Geometry check sheet. Reference: the model listing, model coordinates, mm. A direction names the side the tool comes from. Round coordinates to 2 decimals unless told otherwise and drop trailing zeros. Write each loop counter-clockwise with the first axis right and the second up, starting at its lowest first coordinate (ties: lowest second). Pieces come first, ordered by that corner, then holes. Notation, with made-up numbers: (-15.5, 14) -> (16.5, 14) arc R26 cw to (16.5, 28) -> close; hole circle Ø10 at (-6, 62.5). An arc over 180 degrees is marked (long way). One line per question, with ' | ' between items.
```python
from build123d import *

# Parameters (mm, degrees)
BOSS_EXTRUDE1_DEPTH = 180
SKETCH2_R           = 2.9
CUT_EXTRUDE1_DEPTH  = 4
SKETCH3_R           = 1.7
CUT_EXTRUDE2_DEPTH  = 181.269243078


with BuildPart() as part:
    # Sketch1 → Boss-Extrude1 (new body)
    with BuildSketch(Plane.XY):
        Polygon((9, 6.4), (9, 4.9), (8.2, 4.45), (9, 4), (9, 0), (0, 0), (0, 4), (0.8, 4.45), (0, 4.9), (0, 6.4), align=None)
    extrude(amount=BOSS_EXTRUDE1_DEPTH)

    # Sketch2 → Cut-Extrude1 (cut)
    with BuildSketch(Plane(origin=(0, 6.4, 0), x_dir=(1, 0, 0), z_dir=(0, 1, 0))):
        with Locations(Location((4.5, -170, 0), (0, 0, 270))):
            Circle(SKETCH2_R)
        with Locations(Location((4.5, -150, 0), (0, 0, 270))):
            Circle(SKETCH2_R)
        with Locations(Location((4.5, -130, 0), (0, 0, 270))):
            Circle(SKETCH2_R)
        with Locations(Location((4.5, -110, 0), (0, 0, 270))):
            Circle(SKETCH2_R)
        with Locations(Location((4.5, -90, 0), (0, 0, 270))):
            Circle(SKETCH2_R)
        with Locations(Location((4.5, -70, 0), (0, 0, 270))):
            Circle(SKETCH2_R)
        with Locations(Location((4.5, -50, 0), (0, 0, 270))):
            Circle(SKETCH2_R)
        with Locations(Location((4.5, -30, 0), (0, 0, 270))):
            Circle(SKETCH2_R)
        with Locations(Location((4.5, -10, 0), (0, 0, 270))):
            Circle(SKETCH2_R)
    extrude(amount=-CUT_EXTRUDE1_DEPTH, mode=Mode.SUBTRACT)

    # Sketch3 → Cut-Extrude2 (cut, through all)
    with BuildSketch(Plane(origin=(0, 2.4, 0), x_dir=(1, 0, 0), z_dir=(0, 1, 0))):
        with Locations(Location((4.5, -170, 0), (0, 0, 270))):
            Circle(SKETCH3_R)
        with Locations(Location((4.5, -150, 0), (0, 0, 270))):
            Circle(SKETCH3_R)
        with Locations(Location((4.5, -130, 0), (0, 0, 270))):
            Circle(SKETCH3_R)
        with Locations(Location((4.5, -110, 0), (0, 0, 270))):
            Circle(SKETCH3_R)
        with Locations(Location((4.5, -90, 0), (0, 0, 270))):
            Circle(SKETCH3_R)
        with Locations(Location((4.5, -70, 0), (0, 0, 270))):
            Circle(SKETCH3_R)
        with Locations(Location((4.5, -50, 0), (0, 0, 270))):
            Circle(SKETCH3_R)
        with Locations(Location((4.5, -30, 0), (0, 0, 270))):
            Circle(SKETCH3_R)
        with Locations(Location((4.5, -10, 0), (0, 0, 270))):
            Circle(SKETCH3_R)
    extrude(amount=-CUT_EXTRUDE2_DEPTH, mode=Mode.SUBTRACT)


solid = part.part
```
(1) Access from +Z, -Z, +X, -X, +Y, -Y to the whole of each face (thin tool, end or side, straight path). Record for faces 5 (the cylindrical face through (3.85, 1.22, 131.57)), 6 (the cylindrical face through (5.371, 4.428, 32.766)).
Resolved:
face 5: +Y, -Y | face 6: +Y
(2) Draft check along Z on faces 1 (the flat face through (2.6, 2.4, 70)), 2 (the flat face through (5, 3, 0)), 3 (the flat face through (5, 3, 180)), 4 (the flat face through (2.6, 0, 88.7)). Enter one of: +Z half, -Z half, draft (parallel to the pull), parting line (faces both ways), or undercut.
Resolved:
face 1: undercut | face 2: -Z half | face 3: +Z half | face 4: draft
(3) Sectioned sample at A-A on z = 110. Record the cut outline in (x, y), then the cut area to 3 significant figures.
Resolved:
outline: (0, 0) -> (2.8, 0) -> (2.8, 2.4) -> (1.6, 2.4) -> (1.6, 6.4) -> (0, 6.4) -> (0, 4.9) -> (0.8, 4.45) -> (0, 4) -> close; (6.2, 0) -> (9, 0) -> (9, 4) -> (8.2, 4.45) -> (9, 4.9) -> (9, 6.4) -> (7.4, 6.4) -> (7.4, 2.4) -> (6.2, 2.4) -> close | area: 25.5 mm2
(4) Go/stop test with flat-tipped pins: pin 1 (4 mm diameter, centred on x = 4.5, z = 170, fed in from +Y); pin 2 (1.7 mm diameter, centred on x = 4, z = 30.5, fed in from +Y); pin 3 (3.5 mm diameter, centred on x = 4.5, z = 50, fed in from -Y). Record where each tip stops, or that it passes through.
Resolved:
pin 1: stops at y = 2.4 | pin 2: passes through | pin 3: stops at y = 0
(5) Sectioned sample at B-B on y = 1. Count the separate pieces of the cut face and the enclosed holes in it, then the cut area to 3 significant figures.
Resolved:
separate pieces: 1 | enclosed holes: 9 | area: 1,540 mm2
(6) Material ranges on line 1 (X direction, y = 0.65, z = 130); line 2 (X direction, y = 3.2, z = 30); line 3 (Y direction, x = 3.25, z = 151.5), recorded low to high.
Resolved:
line 1: x = 0 to 2.8, 6.2 to 9 | line 2: x = 0 to 1.6, 7.4 to 9 | line 3: y = 0 to 2.4
